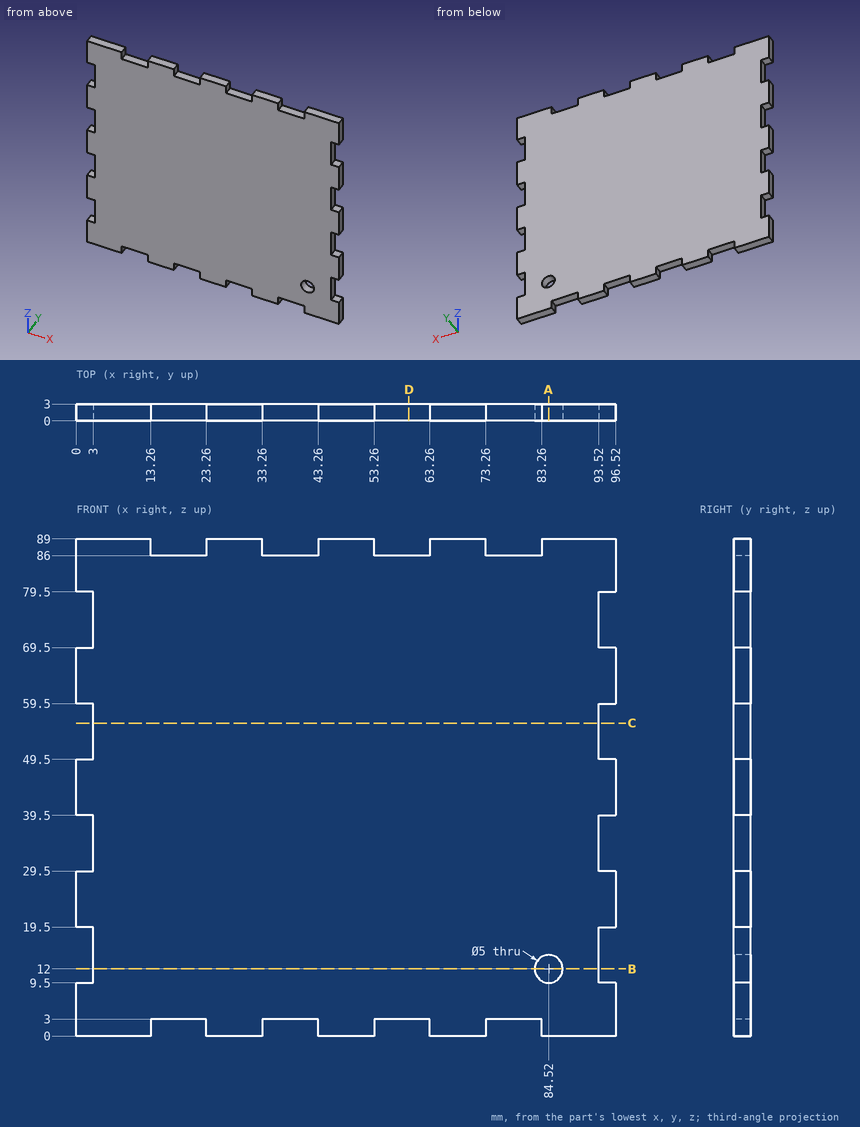
Geometry check sheet. Reference: drawing and pictorial views, mm from the part's lowest x, y, z. Round coordinates to 2 decimals unless told otherwise and drop trailing zeros. Loops run counter-clockwise (first coordinate to the right, second up) from the corner with the lowest first, then second, coordinate; pieces in that order, holes last.
1. Sectioned sample at C-C on z = 56. Record the boundary of the cut face in (x, y), and give its area (3 significant figures).
2. Scan lines: probe 1 along Z at (x, y) = (84.52, 0.65); probe 2 along X at (y, z) = (2.35, 12); probe 3 along X at (y, z) = (1, 18). Record each from-to range of solid material in increasing order.
3. Sectioned sample at A-A on x = 84.52. Record the boundary of the cut face in (y, z), and give its area (3 significant figures).
4. Sectioned sample at B-B on z = 12. Record the boundary of the cut face in (x, y), and give its area (3 significant figures).
5. Gauge pin test, flat end, axial feed: pin 1 Ø1.5 at (y, z) = (1, 14) entering from -X. Record the tip position at first contact, or that the pin passes through.
6. Sectioned sample at D-D on x = 59.5. Record the boundary of the cut face in (y, z), and give its area (3 significant figures).
Recorded:
1. outline: (3, 0) - (93.52, 0) - (93.52, 3) - (3, 3) - close
1. area: 272 mm2
2. probe 1: z = 0 to 9.5, 14.5 to 89
2. probe 2: x = 3 to 82.02, 87.02 to 93.52
2. probe 3: x = 3 to 93.52
3. outline: (0, 0) - (3, 0) - (3, 9.5) - (0, 9.5) - close; (0, 14.5) - (3, 14.5) - (3, 89) - (0, 89) - close
3. area: 252 mm2
4. outline: (3, 0) - (82.02, 0) - (82.02, 3) - (3, 3) - close; (87.02, 0) - (93.52, 0) - (93.52, 3) - (87.02, 3) - close
4. area: 257 mm2
5. pin 1: stops at x = 3
6. outline: (0, 3) - (3, 3) - (3, 86) - (0, 86) - close
6. area: 249 mm2
